Design review of the part shown in the three views and the two pictorial views. Dimensions are in mm from the part's minimum x, y and z. Coordinates: 2 decimals unless noted, no trailing zeros. Write each loop counter-clockwise with the first axis right and the second up, starting at its lowest first coordinate (ties: lowest second). Pieces come first, ordered by that corner, then holes. Notation, with made-up numbers: (38, 6.25) - (73, 6.25) arc R11 cw to (73, 14.25) - close; hole circle Ø5 at (11.5, 36). An arc over 180 degrees is marked (long way). Return JSON: item names as keys, results as strings. Group by question number.
(1) We need section B-B on z = 1.3. State the section outline as (x, y) points.
(2) We need section C-C on x = 80.5. State the section outline as (y, z) points.
(3) We need section A-A on y = 20. State the section outline as (x, z) points, then the cut area to 3 significant figures.
(4) To check wall thickness, follow L1, parallel to Y at x = 88, z = 2.75; L2, parallel to X at y = 200, z = 2.3. State the ranges of each line that lie inside material, in increasing order. Write a range as from..to.
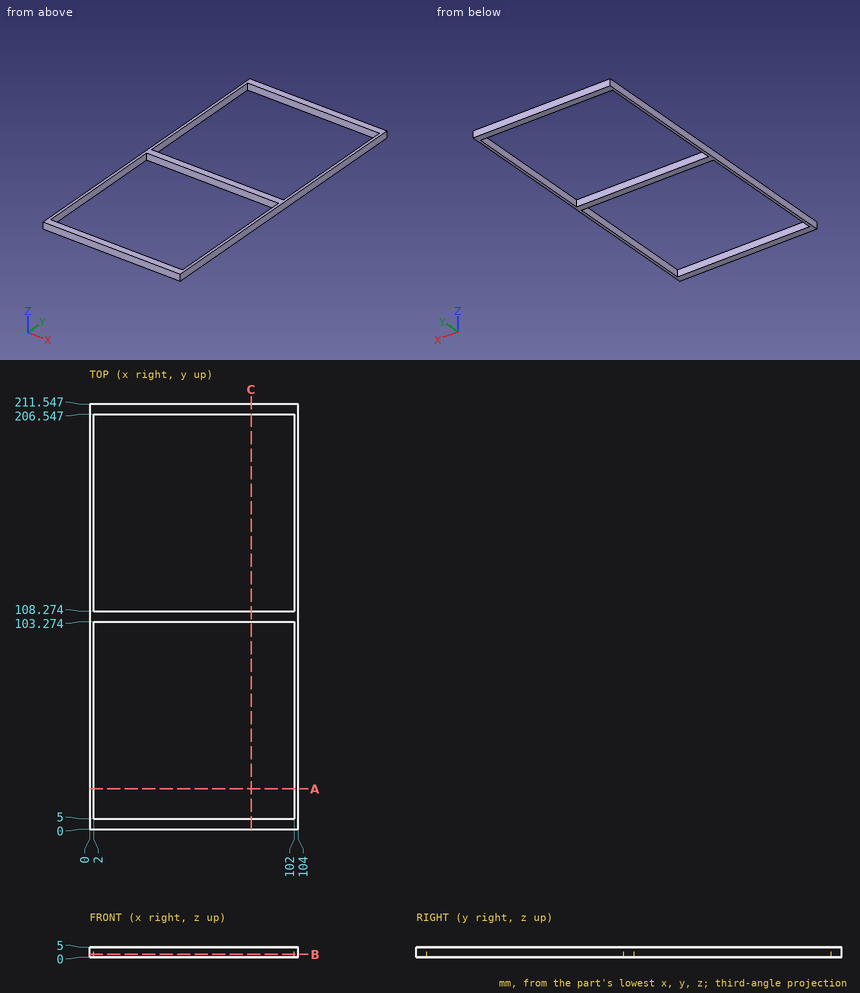
Ans:
{
 "1": {"outline": "(0, 0) - (104, 0) - (104, 211.55) - (0, 211.55) - close; hole (2, 5) - (102, 5) - (102, 103.27) - (2, 103.27) - close; hole (2, 108.27) - (102, 108.27) - (102, 206.55) - (2, 206.55) - close"},
 "2": {"outline": "(0, 0) - (5, 0) - (5, 5) - (0, 5) - close; (103.27, 0) - (108.27, 0) - (108.27, 5) - (103.27, 5) - close; (206.55, 0) - (211.55, 0) - (211.55, 5) - (206.55, 5) - close"},
 "3": {"outline": "(0, 0) - (2, 0) - (2, 5) - (0, 5) - close; (102, 0) - (104, 0) - (104, 5) - (102, 5) - close", "area": "20.0 mm²"},
 "4": {"L1": "0..5, 103.27..108.27, 206.55..211.55", "L2": "0..2, 102..104"}
}
